Autodesk Inventor part; units mm, degrees
ref_plane "Work Plane1" through (-4, 0, -155) normal (0, 0, -1) x (-1, 0, 0)
ref_plane "YZ Plane" through (0, 0, 0) normal (1, 0, 0) x (0, 1, 0)
ref_plane "XZ Plane" through (0, 0, 0) normal (0, 1, 0) x (-1, 0, 0)
sketch "Sketch1" plane through (0, 0, 0) normal (0, 1, 0) x (-1, 0, 0)
  line L0 (0, 0) -> (52, 0)
  line L1 (52, 0) -> (52, -129)
  line L2 (52, -129) -> (0, -129)
  line L3 (0, -129) -> (0, 0)
  dimension "d0" = 52
  dimension "d1" = 129
extrude "Extrusion1" add sketch "Sketch1" along normal blind 39
fillet "Fillet1" radius 4 4 edges at (0, 19.5, 0) (0, 19.5, -129) (-52, 19.5, 0) (-52, 19.5, -129)
sketch "Sketch2" plane through (-48, 0, 0) normal (0, 0, 1) x (1, 0, 0)
  line L0 (44, 39) -> (0, 39)
  line L1 (0, 39) -> (0, 31)
  line L2 (0, 39) -> (0, 0)
  line L3 (0, 31) -> (23, 31)
  line L4 (23, 31) -> (23, 13)
  line L5 (23, 13) -> (0, 13)
  line L6 (0, 13) -> (0, 31)
  point P0 (48, 0)
  dimension "d5" = 8
  dimension "d6" = 23
  dimension "d7" = 18
extrude "Extrusion2" cut sketch "Sketch2" against normal blind 5
sketch "Sketch3" plane through (-4, 0, -129) normal (0, 0, -1) x (-1, 0, 0)
  line L0 (0, 39) -> (44, 39)
  line L1 (44, 39) -> (44, 36)
  line L2 (44, 39) -> (44, 0)
  line L3 (44, 36) -> (41, 36)
  line L4 (41, 36) -> (36.9695, 31.9695)
  line L5 (41, 36) -> (46.7, 36) construction
  circle A0 centre (36.9695, 31.9695) radius 5.7
  point P0 (-4, 0)
  dimension "d10" = 3
  dimension "d11" = 3
  dimension "d12" = 5.7
  dimension "d13" = 135
ref_plane "Work Plane1" through (-4, 0, -155) normal (0, 0, -1) x (-1, 0, 0)
sketch "Sketch4" plane through (-4, 0, -155) normal (0, 0, -1) x (-1, 0, 0)
  line L0 (0, 39) -> (44, 39)
  line L1 (44, 39) -> (44, 36)
  line L2 (44, 39) -> (44, 0)
  line L3 (44, 36) -> (41, 36)
  line L4 (41, 36) -> (36.9695, 31.9695)
  line L5 (41, 36) -> (46.7, 36) construction
  circle A0 centre (36.9695, 31.9695) radius 4.25
  point P0 (-4, 0)
  dimension "d15" = 3
  dimension "d16" = 3
  dimension "d17" = 5.7
  dimension "d18" = 135
  dimension "d19" = 8.5
loft "Loft1" add profiles "Sketch3", "Sketch4"
properties part number "NucPowerBrick"
For this review, take the finished solid that the model builds, in its own axes (mm). A direction names the side the tool comes from. Coordinates: 2 decimals unless noted, no trailing zeros. Write each loop counter-clockwise with the first axis right and the second up, starting at its lowest first coordinate (ties: lowest second). Pieces come first, ordered by that corner, then holes.
(1) Tool access review of faces 4 (the face through (-25, 22, -2)), 5 (the face through (-1.203, 19.773, -1.141)): name each direction out of +Z, -Z, +X, -X, +Y, -Y from which nothing blocks a thin tool from reaching the whole face with its end or side.
(2) Add section A-A on y = 3. Give the boundary of the cut face in (x, z).
(3) Wall thickness on probe 1 along Z at (x, y) = (-46, 18.5); probe 2 along Z at (x, y) = (-19, 11.5); probe 3 along Y at (x, z) = (-40.5, -134.5): over which ranges is each line inside the solid? List them lowest first.
(4) For pin 1 Ø5.5 at (x, y) = (-38, 26) entering from +Z; pin 2 Ø1.5 at (y, z) = (19.5, -2) entering from +X, all flat-tipped, find the tip position at first contact; note any pin that passes through.
(5) Add section C-C on y = 19.5. Give the boundary of the cut face in (x, z), then the cut area to 3 significant figures.
(6) Add section B-B on x = -27.5. Give the boundary of the cut face in (y, z).
(7) Add section D-D on x = -9. Give the boundary of the cut face in (y, z), then the cut area to 3 significant figures.
(8) The part is to be moulded in two halves that separate along Y. For faces 1 (the face through (-26, 0, -64)), 2 (the face through (-37, 22, -5)), 3 (the face through (-52, 19, -64)), say which applies: +Y half, -Y half, draft (parallel to the pull), parting line (faces both ways), or undercut.
Answer sheet:
1. face 4: +Z
1. face 5: +Z, +X, +Y, -Y
2. outline: (-52, -125) arc R4 ccw to (-48, -129) - (-4, -129) arc R4 ccw to (0, -125) - (0, -4) arc R4 ccw to (-4, 0) - (-48, 0) arc R4 ccw to (-52, -4) - close
3. probe 1: z = -129 to -5
3. probe 2: z = -129 to 0
3. probe 3: y = 26.6 to 37.34
4. pin 1: stops at z = -5
4. pin 2: stops at x = -0.2
5. outline: (-52, -125) arc R4 ccw to (-48, -129) - (-4, -129) arc R4 ccw to (0, -125) - (0, -4) arc R4 ccw to (-4, 0) - (-25, 0) - (-25, -5) - (-48, -5) - (-48, 0) arc R4 ccw to (-52, -4) - close
5. area: 6,580 mm2
6. outline: (0, -129) - (39, -129) - (39, 0) - (31, 0) - (31, -5) - (13, -5) - (13, 0) - (0, 0) - close
7. outline: (0, -129) - (39, -129) - (39, 0) - (0, 0) - close
7. area: 5,030 mm2
8. face 1: -Y half
8. face 2: undercut
8. face 3: draft
